Verification items for the finished model (mm, model axes). A direction names the side the tool comes from. Give positions to 0.01 mm unless a question says otherwise; leave off trailing zeros. Order: outer loops, then holes, each group sorted by start corner. A loop starts at its lowest first (then second) coordinate and runs counter-clockwise, first axis right, second up.
(1) Sectioned sample at A-A on y = 15.06. Record the cut outline in (x, z) (3 decimals), plus the area to 4 significant figures.
(2) Sectioned sample at B-B on z = -15. Count the separate pieces of the cut face and the enclosed holes in it, plus the area to 3 significant figures.
(3) Sectioned sample at D-D on x = 6. Record the cut outline in (y, z).
(4) Gauge pin test, flat ends, axial feed: pin 1 (5 mm diameter, centred on y = 38, z = -21.5, fed in from -X); pin 2 (4 mm diameter, centred on y = 23.56, z = -15, fed in from -X); pin 3 (7.5 mm diameter, centred on y = 7.5, z = -14.5, fed in from -X); pin 4 (9 mm diameter, centred on x = -2.5, z = -16, fed in from -Y). Record the tip position at first contact, or that the pin passes through.
(5) Sectioned sample at C-C on x = 23.5. Record the cut outline in (y, z) (3 decimals).
(6) Mould release check, pull along Y, two halves, no side actions. Record for faces 1 (the face through (3, 152, -15)), 2 (the face through (25.07, 15.171, -12.477)), 3 (the face through (25, -7, -21.975)): pulls with the +Y half, pulls with the -Y half, needs draft (parallel to the pull), parting line crosses it, or undercut.
(7) Access from +Z, -Z, +X, -X, +Y, -Y to the whole of each face (thin tool, end or side, straight path). Record for faces 4 (the face through (15, 0, -3)), 5 (the face through (10, 15, -4.95)), 6 (the face through (1, 138, -15)), 7 (the face through (-4, 100, -15)), 8 (the face through (21.035, 7.973, -10.515)).
(8) Scan lines: L1, parallel to Y at x = 21.4, z = -15 (1 decimal); L2, parallel to Z at x = 27.5, y = 23.56; L3, parallel to Z at x = 9, y = 16.5. Record each from-to range of solid material in increasing order.
Autodesk Inventor part; units mm, degrees
ref_plane "YZ Plane" through (0, 0, 0) normal (1, 0, 0) x (0, 1, 0)
ref_plane "XZ Plane" through (0, 0, 0) normal (0, 1, 0) x (-1, 0, 0)
ref_plane "XY Plane" through (0, 0, 0) normal (0, 0, 1) x (1, 0, 0)
sketch "Sketch1" plane through (0, 0, 0) normal (0, 0, 1) x (1, 0, 0)
  line L0 (0, 0) -> (25, 0)
  line L1 (25, 0) -> (25, 40)
  line L2 (25, 40) -> (0, 40)
  line L3 (0, 40) -> (0, 0)
  dimension "d1" = 25
  dimension "d2" = 40
  dimension "d3" = 25
extrude "Extrusion1" add sketch "Sketch1" against normal blind 30
sketch "Sketch2" plane through (25, 0, 0) normal (1, 0, 0) x (0, 0, -1)
  line L0 (0, 0) -> (30, 0)
  circle A0 centre (15, 6.56) radius 2.46
extrude "Extrusion2" cut sketch "Sketch2" against normal blind 30
sketch "Sketch3" plane through (0, 0, 0) normal (-1, 0, 0) x (0, 0, 1)
  line L0 (0, 0) -> (-30, 0)
  line L1 (-25.05, 0) -> (-4.95, 0)
  line L2 (-4.95, 0) -> (-4.95, 33.12)
  line L3 (-4.95, 33.12) -> (-25.05, 33.12)
  line L4 (-25.05, 33.12) -> (-25.05, 0)
  dimension "d11" = 20.1
extrude "Extrusion3" cut sketch "Sketch3" against normal blind 20
sketch "Sketch4" plane through (0, 0, 0) normal (0, -1, 0) x (1, 0, 0)
  line L0 (20, -4.95) -> (20, -25.05)
  line L1 (20, -15) -> (25, -15)
  line L2 (25, 0) -> (25, -30)
  line L3 (20, -8.025) -> (25, -8.025)
  line L4 (25, -8.025) -> (25, -21.975)
  line L5 (25, -21.975) -> (20, -21.975)
  line L6 (20, -21.975) -> (20, -8.025)
  line L7 (20, -8.025) -> (25, -21.975) construction
  line L8 (25, -8.025) -> (20, -21.975) construction
  line L9 (25, -12.54) -> (25, -17.46)
  point P0 (0, 0)
  point P1 (22.5, -15)
  dimension "d14" = 13.95
extrude "Extrusion4" add sketch "Sketch4" along normal blind 15
sketch "Sketch5" plane through (20, 0, 0) normal (-1, 0, 0) x (0, 0, 1)
  circle A0 centre (-15, 6.56) radius 2.46
  circle A1 centre (-15, 6.56) radius 4.7025
  circle A2 centre (-15, 6.56) radius 2.46
  circle A3 centre (-15, 6.56) radius 2.46
  point P0 (0, 0)
  dimension "d17" = 9.405
extrude "Extrusion5" cut sketch "Sketch5" against normal blind 2.1
sketch "Sketch6" plane through (25, 0, 0) normal (1, 0, 0) x (0, 0, -1)
  circle A0 centre (15, 6.56) radius 4.7025
  line L0 (15, 6.56) -> (15, 23.56)
  circle A1 centre (15, 23.56) radius 2.46
  point P0 (0, 0)
  dimension "d20" = 17
  dimension "d21" = 4.92
extrude "Extrusion6" cut sketch "Sketch6" against normal blind 10 contours A1
sketch "Sketch7" plane through (20, 0, 0) normal (-1, 0, 0) x (0, 0, 1)
  circle A0 centre (-15, 23.56) radius 2.46
  circle A1 centre (-15, 23.56) radius 4.7025
  point P0 (0, 0)
  dimension "d24" = 9.405
extrude "Extrusion7" cut sketch "Sketch7" against normal blind 2.1
sketch "Sketch9" plane through (25, 0, 0) normal (1, 0, 0) x (0, 0, -1)
  circle A0 centre (15, 6.56) radius 2.46
  circle A1 centre (15, 6.56) radius 2.46
  circle A2 centre (15, 23.56) radius 2.46
  circle A3 centre (15, 23.56) radius 2.46
  line L0 (30, 40) -> (30, 0)
  line L1 (30, 0) -> (30, 40)
  line L2 (30, 40) -> (0, 40)
  line L3 (0, 40) -> (0, 0)
  line L4 (0, 0) -> (8.025, 0)
  line L5 (21.975, 0) -> (21.975, -15)
  line L6 (21.975, -15) -> (8.025, -15)
  line L7 (8.025, -15) -> (8.025, 0)
  line L8 (0, 0) -> (8.025, 0)
  line L9 (21.975, 0) -> (30, 0)
extrude "Extrusion8" add sketch "Sketch9" along normal blind 5
sketch "Sketch10" plane through (0, 40, 0) normal (0, 1, 0) x (1, 0, 0)
  line L0 (0, 30) -> (30, 30)
  line L1 (30, 0) -> (0, 0)
  line L2 (0, 30) -> (30, 30)
  line L3 (30, 30) -> (30, 0)
  line L4 (30, 0) -> (0, 0)
  line L5 (0, 0) -> (0, 30)
extrude "Extrusion9" add sketch "Sketch10" along normal blind 30
sketch "Sketch12" plane through (30, 0, 0) normal (1, 0, 0) x (0, 0, -1)
  circle A0 centre (15, 6.56) radius 2.46
  line L0 (15, 6.56) -> (15, 15.06)
  circle A1 centre (15, 15.06) radius 2.525
  point P0 (0, 0)
  dimension "d31" = 8.5
  dimension "d33" = 5.05
extrude "Extrusion10" cut sketch "Sketch12" against normal blind 30 contours A1
sketch "Sketch14" plane through (0, 0, 0) normal (0, 0, 1) x (1, 0, 0)
  line L0 (30, 70) -> (0, 70)
  line L1 (0, 100) -> (-8, 100)
  line L2 (30, 0) -> (30, 70)
  line L3 (30, 118) -> (30, 70)
  line L4 (30, 105) -> (30, 100)
  line L5 (0, 70) -> (30, 70)
  line L6 (0, 70) -> (0, 100)
  line L7 (30, 122.5) -> (30, 118)
  line L8 (-2, 150) -> (-8, 152)
  line L9 (-2, 102) -> (-8, 100)
  line L10 (-2, 102) -> (4, 126)
  line L11 (4, 126) -> (-2, 150)
  line L12 (-8, 152) -> (15, 152)
  line L13 (30, 137) -> (15, 152)
  line L14 (30, 122.5) -> (30, 137)
  point P0 (0, 0)
  dimension "d47" = 30
extrude "Extrusion12" add sketch "Sketch14" against normal blind 30
sketch "Sketch15" plane through (0, 0, -25.05) normal (-1, 0, 0) x (0, 0, 1)
  line L0 (0, 33.12) -> (20.1, 33.12)
  line L1 (20.1, 33.12) -> (20.1, 0)
  line L2 (0, 33.12) -> (20.1, 33.12)
  line L3 (20.1, 33.12) -> (20.1, 31.1)
  line L4 (20.1, 31.1) -> (0, 31.1)
  line L5 (0, 31.1) -> (0, 33.12)
  point P0 (25.05, 0)
  dimension "d57" = 2.02
extrude "Extrusion13" add sketch "Sketch15" against normal blind 20
sketch "Sketch25" plane through (0, 0, 0) normal (0, 0, 1) x (1, 0, 0)
  point P0 (0, 0)
properties part number "48mm_x_30mm"
Ans:
1. outline: (0, -30) - (30, -30) - (30, -17.525) - (20, -17.525) - (20, -25.05) - (0, -25.05) - close; (0, -4.95) - (20, -4.95) - (20, -12.475) - (30, -12.475) - (30, 0) - (0, 0) - close
1. area: 447.5 mm2
2. separate pieces: 4
2. enclosed holes: 0
2. area: 3,780 mm2
3. outline: (0, -30) - (152, -30) - (152, 0) - (0, 0) - (0, -4.95) - (31.1, -4.95) - (31.1, -25.05) - (0, -25.05) - close
4. pin 1: stops at x = 0
4. pin 2: passes through
4. pin 3: stops at x = 20
4. pin 4: stops at y = 31.1
5. outline: (-15, -21.975) - (0, -21.975) - (0, -30) - (143.5, -30) - (143.5, 0) - (0, 0) - (0, -8.025) - (-15, -8.025) - close; hole circle Ø4.92 at (6.56, -15); hole circle Ø5.05 at (15.06, -15); hole circle Ø4.92 at (23.56, -15)
6. face 1: pulls with the +Y half
6. face 2: undercut
6. face 3: needs draft
7. face 4: +Z, +X, -X, -Y
7. face 5: -X, -Y
7. face 6: +Z, -Z, -X
7. face 7: +Z, -Z, -X, -Y
7. face 8: -X
8. L1: y = -15 to 1.9, 11.3 to 12.5, 17.6 to 18.9, 28.3 to 145.6
8. L2: z = -30 to -17.46, -12.54 to 0
8. L3: z = -30 to -25.05, -4.95 to 0
